The model under review builds one solid part; all positions refer to its coordinate system, in mm. A direction names the side the tool comes from. Give positions to 0.01 mm unless a question says otherwise; leave off trailing zeros. Order: outer loops, then holes, each group sorted by start corner. A loop starts at its lowest first (then second) coordinate and runs counter-clockwise, first axis right, second up. Notation, with made-up numbers: (-19.5, 42.25) - (0.5, 42.25) arc R18 cw to (0.5, 69.25) - close; hole circle Ø4 at (-24.5, -5.5). An arc over 180 degrees is marked (long way). Put each result on its own line as item: value.
```python
from build123d import *

# Parameters (mm, degrees)
SKETCH1_W           = 20.57
SKETCH1_H           = 15.8
BOSS_EXTRUDE1_DEPTH = 15.24
FILLET1_R           = 4
SKETCH2_R           = 1.6
BOSS_EXTRUDE2_DEPTH = 3.6
SKETCH2_4_R         = 0.45
BOSS_EXTRUDE3_DEPTH = 4
SKETCH2_5_R         = 0.45
BOSS_EXTRUDE4_DEPTH = 4
LPATTERN1_COUNT     = 3
LPATTERN1_PITCH     = 2.54
LPATTERN1_COL_COUNT = 2
LPATTERN1_COL_PITCH = 2.54
LPATTERN2_COUNT     = 2
LPATTERN2_PITCH     = 2.54
LPATTERN2_COL_COUNT = 3
LPATTERN2_COL_PITCH = 2.54


with BuildPart() as part:
    # Sketch1 → Boss-Extrude1 (new body)
    with BuildSketch(Plane.XY):
        Rectangle(SKETCH1_W, SKETCH1_H)
    extrude(amount=BOSS_EXTRUDE1_DEPTH)

    # Fillet1
    fillet1_edges = [part.edges().sort_by_distance(p)[0] for p in [
        (10.285, 7.9, 7.62),
    ]]
    fillet(fillet1_edges, radius=FILLET1_R)

    # Sketch2 → Boss-Extrude2 (add)
    with BuildSketch(Plane.XZ.offset(7.9)):
        with Locations(Location((0.125, 1.905, 0), (0, 0, 90))):
            Circle(SKETCH2_R)
        with Locations(Location((0.125, 13.335, 0), (0, 0, 90))):
            Circle(SKETCH2_R)
    extrude(amount=BOSS_EXTRUDE2_DEPTH)

    # Sketch2_4 → Boss-Extrude3 (add)
    with BuildSketch(Plane.XZ.offset(7.9)):
        with Locations(Location((6.475, 6.985, 0), (0, 0, 90))):
            Circle(SKETCH2_4_R)
    boss_extrude3 = extrude(amount=BOSS_EXTRUDE3_DEPTH)

    # Sketch2_5 → Boss-Extrude4 (add)
    with BuildSketch(Plane.XZ.offset(7.9)):
        with Locations(Location((9.015, 8.255, 0), (0, 0, 90))):
            Circle(SKETCH2_5_R)
    boss_extrude4 = extrude(amount=BOSS_EXTRUDE4_DEPTH)

    # LPattern1: Boss-Extrude4 ×3
    with Locations(*[(0, 0, -i * LPATTERN1_PITCH) for i in range(1, LPATTERN1_COUNT)]):
        add(boss_extrude4)

    # LPattern1 col: Boss-Extrude4 ×2
    with Locations(*[(0, 0, i * LPATTERN1_COL_PITCH) for i in range(1, LPATTERN1_COL_COUNT)]):
        add(boss_extrude4)

    # LPattern2: Boss-Extrude3 ×2
    with Locations(*[(0, 0, -i * LPATTERN2_PITCH) for i in range(1, LPATTERN2_COUNT)]):
        add(boss_extrude3)

    # LPattern2 col: Boss-Extrude3 ×3
    with Locations(*[(0, 0, i * LPATTERN2_COL_PITCH) for i in range(1, LPATTERN2_COL_COUNT)]):
        add(boss_extrude3)


solid = part.part
```
(1) Take a section at C-C, the plane x = 1. Write out the cut boundary in (y, z), then the cut area to 3 significant figures.
The answers:
outline: (-11.5, 0.57) - (-7.9, 0.57) - (-7.9, 0) - (7.9, 0) - (7.9, 15.24) - (-7.9, 15.24) - (-7.9, 14.67) - (-11.5, 14.67) - (-11.5, 12) - (-7.9, 12) - (-7.9, 3.24) - (-11.5, 3.24) - close
area: 260 mm^2
(2) Take a section at A-A, the plane y = -9. Count the separate pieces of the cut face and the enclosed holes in it, then the cut area to 3 significant figures.
The answers:
separate pieces: 10
enclosed holes: 0
area: 21.2 mm^2
(3) The part is to be moulded in two halves that separate along Z. For faces 4 (the cylindrical face through (6.65, -9.87, 12.48)), 5 (the flat face through (0, 0, 15.24)), 6 (the flat face through (0, 0, 0)), 7 (the flat face through (6.5, -11.9, 12.1)), say which applies: pulls with the +Z half, pulls with the -Z half, needs draft (parallel to the pull), parting line crosses it, or undercut.
The answers:
face 4: undercut
face 5: pulls with the +Z half
face 6: pulls with the -Z half
face 7: needs draft
(4) Take a section at D-D, the plane z = 1.5. Write out the cut boundary in (x, y) (3 decimals).
The answers:
outline: (-10.285, -7.9) - (-1.423, -7.9) - (-1.423, -11.5) - (1.673, -11.5) - (1.673, -7.9) - (10.285, -7.9) - (10.285, 3.9) arc R4 ccw to (6.285, 7.9) - (-10.285, 7.9) - close
(5) For faces 1 (the cylindrical face through (6.65, -9.87, 7.4)), 2 (the flat face through (9, -11.9, 3)), 3 (the flat face through (0, -11.5, 2)), list the 3-axis set-ups (+Z, -Z, +X, -X, +Y, -Y) from which the entire face can be reached by the end or side of a thin tool; tool diameter is ignored.
The answers:
face 1: -Y
face 2: +Z, -Z, +X, -X, -Y
face 3: +Z, -Z, -X, -Y
(6) Wall thickness on L1, parallel to Z at x = 9, y = -10.25; L2, parallel to Y at x = -4, z = 14.5; L3, parallel to Y at x = 1.5, z = 12.75: over which ranges is each line inside the solid? List them lowest first.
The answers:
L1: 2.73 to 3.62, 5.27 to 6.16, 7.81 to 8.7, 10.35 to 11.24
L2: -7.9 to 7.9
L3: -11.5 to 7.9
(7) Take a section at B-B, the plane z = 5.75. Write out the cut boundary in (x, y) (3 decimals), then the cut area to 3 significant figures.
The answers:
outline: (-10.285, -7.9) - (8.566, -7.9) - (8.566, -11.9) - (9.464, -11.9) - (9.464, -7.9) - (10.285, -7.9) - (10.285, 3.9) arc R4 ccw to (6.285, 7.9) - (-10.285, 7.9) - close
area: 325 mm^2
(8) Clearance check with flat-ended pins moving along their axes: pin 1 Ø1 at (x, y) = (6, -8.5) entering from -Z (3 decimals); pin 2 Ø2.5 at (x, z) = (-0.5, 14) entering from -Y. State where each tip first meets the part, or that it passes through.
The answers:
pin 1: z = 3.995
pin 2: y = -11.5
